from build123d import *

# Parameters (mm, degrees)
SKETCH1_W                        = 50.8
SKETCH1_H                        = 6.35
EXTRUDE1_DEPTH                   = 97.8408
F_1_4_CLEARANCE_HOLE1_AT_2_COUNT = 2
F_1_4_CLEARANCE_HOLE1_AT_2_PITCH = 44.45


with BuildPart() as part:
    # Sketch1 → Extrude1 (new body)
    with BuildSketch(Plane.XY):
        Rectangle(SKETCH1_W, SKETCH1_H)
    extrude(amount=EXTRUDE1_DEPTH)

    # Sketch4 → 3/8 Clearance Hole1 (revolve, cut)
    with BuildSketch(Plane(origin=(12.7, 3.175, 85.1408), x_dir=(0, 0, 1), z_dir=(1, 0, 0))):
        Polygon((0, 0), (0, 19.031479155), (5.0419, 16.002), (5.0419, 0), align=None)
    f_3_8_clearance_hole1 = revolve(axis=Axis((12.7, 9.525, 85.1408), (0, -1, 0)), mode=Mode.SUBTRACT)

    # Sketch5 → 1/4 Clearance Hole1 (revolve, cut)
    with BuildSketch(Plane(origin=(12.7, 3.175, 57.15), x_dir=(0, 0, 1), z_dir=(1, 0, 0))):
        Polygon((0, 0), (0, 18.147817477), (3.57124, 16.002), (3.57124, 0), align=None)
    f_1_4_clearance_hole1 = revolve(axis=Axis((12.7, 9.525, 57.15), (0, -1, 0)), mode=Mode.SUBTRACT)

    # 1/4 Clearance Hole1 at 2: 1/4 Clearance Hole1 ×2
    with Locations(*[(0, 0, -i * F_1_4_CLEARANCE_HOLE1_AT_2_PITCH) for i in range(1, F_1_4_CLEARANCE_HOLE1_AT_2_COUNT)]):
        add(f_1_4_clearance_hole1, mode=Mode.SUBTRACT)

    # Mirror1: 3/8 Clearance Hole1, 1/4 Clearance Hole1 across plane
    add(f_3_8_clearance_hole1.mirror(Plane(origin=(0, 0, 0), x_dir=(0, 0, 1), z_dir=(1, 0, 0))), mode=Mode.SUBTRACT)
    add(f_1_4_clearance_hole1.mirror(Plane(origin=(0, 0, 0), x_dir=(0, 0, 1), z_dir=(1, 0, 0))), mode=Mode.SUBTRACT)

    # Mirror1 copy 1 sketch → Mirror1 copy 1 (revolve, cut)
    with BuildSketch(Plane(origin=(-12.7, 3.175, 12.7), x_dir=(0, 0, 1), z_dir=(-1, 0, 0))):
        Polygon((0, 0), (0, -18.147817477), (3.57124, -16.002), (3.57124, 0), align=None)
    revolve(axis=Axis((-12.7, 9.525, 12.7), (0, 1, 0)), mode=Mode.SUBTRACT)


solid = part.part
Verification items for the finished model (mm, model axes). Give positions to 0.01 mm unless a question says otherwise; leave off trailing zeros. Loops run counter-clockwise (first coordinate to the right, second up) from the corner with the lowest first, then second, coordinate; pieces in that order, holes last. Notation, with made-up numbers: (46.25, 28) - (63.25, 28) arc R18 ccw to (63.25, 46) - close; hole circle Ø1 at (-16, 75.5). An arc over 180 degrees is marked (long way). Write item = value, one per line. Start each with the question number.
Q1. Cross-section at B-B, the plane z = 12.7. Enter the section's corners in (x, y) (3 decimals), and give its area (3 significant figures).
Q2. Thickness scan on line 1 (Z direction, x = 12.7, y = -1.5); line 2 (X direction, y = 0.5, z = 12.7); line 3 (Z direction, x = -12, y = -1.5). Record the ranges inside material, lowest first.
Q3. Cross-section at A-A, the plane x = 12.7. Enter the section's corners in (y, z) (3 decimals).
Q4. Cross-section at C-C, the plane y = 1.25. Enter the section's corners in (x, z).
Q5. Mould release check, pull along Z, two halves, no side actions. Record for faces 1 (the face through (0, 0, 97.841)), 2 (the face through (12.543, 0.044, 53.582)), 3 (the face through (25.4, 0, 48)): released by +Z, released by -Z, zero draft, split by the parting line, or undercut.
Answer key:
q1.outline = (-25.4, -3.175) - (-16.271, -3.175) - (-16.271, 3.175) - (-25.4, 3.175) - close; (-9.129, -3.175) - (9.129, -3.175) - (9.129, 3.175) - (-9.129, 3.175) - close; (16.271, -3.175) - (25.4, -3.175) - (25.4, 3.175) - (16.271, 3.175) - close
q1.area = 232 mm^2
q2.line_1 = 0 to 9.13, 16.27 to 53.58, 60.72 to 80.1, 90.18 to 97.84
q2.line_2 = -25.4 to -16.27, -9.13 to 9.13, 16.27 to 25.4
q2.line_3 = 0 to 9.2, 16.2 to 53.65, 60.65 to 80.15, 90.13 to 97.84
q3.outline = (-3.175, 0) - (3.175, 0) - (3.175, 9.129) - (-3.175, 9.129) - close; (-3.175, 16.271) - (3.175, 16.271) - (3.175, 53.579) - (-3.175, 53.579) - close; (-3.175, 60.721) - (3.175, 60.721) - (3.175, 80.099) - (-3.175, 80.099) - close; (-3.175, 90.183) - (3.175, 90.183) - (3.175, 97.841) - (-3.175, 97.841) - close
q4.outline = (-25.4, 0) - (25.4, 0) - (25.4, 97.84) - (-25.4, 97.84) - close; hole circle Ø10.08 at (-12.7, 85.14); hole circle Ø7.14 at (-12.7, 12.7); hole circle Ø7.14 at (-12.7, 57.15); hole circle Ø10.08 at (12.7, 85.14); hole circle Ø7.14 at (12.7, 12.7); hole circle Ø7.14 at (12.7, 57.15)
q5.face_1 = released by +Z
q5.face_2 = undercut
q5.face_3 = zero draft
